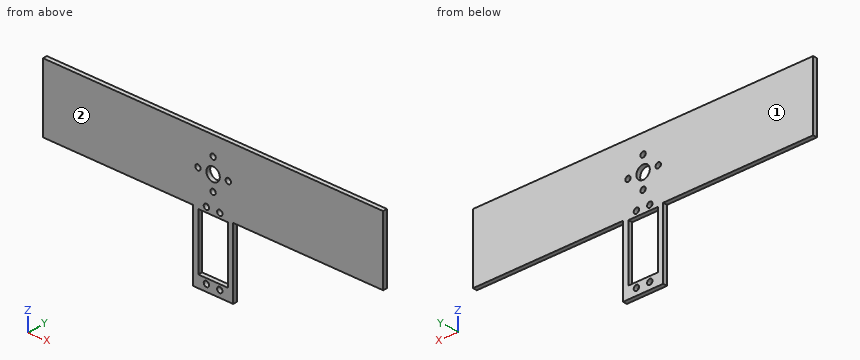
from build123d import *

# Parameters (mm, degrees)
SKETCH1_R           = 2
SKETCH1_R_2         = 5
BOSS_EXTRUDE1_DEPTH = 3.175


with BuildPart() as part:
    # Sketch1 → Boss-Extrude1 (new body)
    with BuildSketch(Plane(origin=(0, 0, 0), x_dir=(1, 0, 0), z_dir=(0, 1, 0))):
        Polygon((254, 0), (142, 0), (142, 52), (112, 52), (112, 0), (0, 0), (0, -50.8), (254, -50.8), align=None)
        with Locations(Location((127, -36.713708499, 0), (0, 0, 270))):
            Circle(SKETCH1_R, mode=Mode.SUBTRACT)
        with Locations(Location((115.686291501, -25.4, 0), (0, 0, 270))):
            Circle(SKETCH1_R, mode=Mode.SUBTRACT)
        with Locations(Location((127, -25.4, 0), (0, 0, 270))):
            Circle(SKETCH1_R_2, mode=Mode.SUBTRACT)
        with Locations(Location((138.313708499, -25.4, 0), (0, 0, 270))):
            Circle(SKETCH1_R, mode=Mode.SUBTRACT)
        with Locations(Location((122, -2.6025933, 0), (0, 0, 270))):
            Circle(SKETCH1_R, mode=Mode.SUBTRACT)
        with Locations(Location((127, -14.086291501, 0), (0, 0, 270))):
            Circle(SKETCH1_R, mode=Mode.SUBTRACT)
        with Locations(Location((132, -2.6025933, 0), (0, 0, 270))):
            Circle(SKETCH1_R, mode=Mode.SUBTRACT)
        Polygon((138, 1.1474067), (127, 1.1474067), (116, 1.1474067), (116, 43.1474067), (127, 43.1474067), (138, 43.1474067), align=None, mode=Mode.SUBTRACT)
        with Locations(Location((122, 46.8974067, 0), (0, 0, 270))):
            Circle(SKETCH1_R, mode=Mode.SUBTRACT)
        with Locations(Location((132, 46.8974067, 0), (0, 0, 270))):
            Circle(SKETCH1_R, mode=Mode.SUBTRACT)
    extrude(amount=BOSS_EXTRUDE1_DEPTH)


solid = part.part
Part model, mm, in its own coordinate system. Face numbers are marked on the shaded views. Round coordinates to 2 decimals unless told otherwise and drop trailing zeros. Write each loop counter-clockwise with the first axis right and the second up, starting at its lowest first coordinate (ties: lowest second). Pieces come first, ordered by that corner, then holes. Notation, with made-up numbers: M 40.25,88 L 95.25,88 A5 ccw 95.25,92 Z; hole C -7,62.25 d3. An arc over 180 degrees is marked long. Return JSON: item names as keys, results as strings. Group by question number.
(1) Saw through at A-A on y = 2.05. Count the separate pieces of the cut face and the enclosed holes in it, then the cut area to 3 significant figures.
(2) Saw through at B-B on x = 33.5. Write the cut outline in (y, z) (3 decimals).
(3) Drill centre lines: probe 1 along X at (y, z) = (1.15, 25.4); probe 2 along X at (y, z) = (0.2, -37.5); probe 3 along X at (y, z) = (2.8, 30). Where is each one in solid material? Low to high.
(4) Pin check, flat tips, straight feed: pin 1 Ø1.6 at (y, z) = (1, -21) entering from -X; pin 2 Ø1 at (y, z) = (2, -26) entering from +X. Stop position of each tip, or through.
(5) Two-plate mould, pull along Y, no slides. Class the marked faces 1 and 2: +Y half, -Y half, draft (parallel to the pull), parting line (faces both ways), or undercut.
Returned:
{
 "1": {"separate pieces": "1", "enclosed holes": "10", "area": "13,400 mm²"},
 "2": {"outline": "M 0,0 L 3.175,0 L 3.175,50.8 L 0,50.8 Z"},
 "3": {"probe 1": "0 to 113.69, 117.69 to 122, 132 to 136.31, 140.31 to 254", "probe 2": "112 to 116, 138 to 142", "probe 3": "0 to 125.04, 128.96 to 254"},
 "4": {"pin 1": "x = 112", "pin 2": "x = 142"},
 "5": {"face 1": "+Y half", "face 2": "-Y half"}
}
